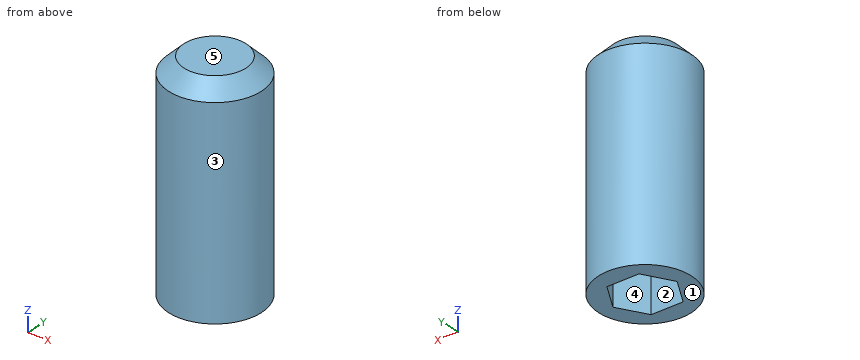
Autodesk Inventor part; units mm, degrees
ref_plane "YZ Plane" through (0, 0, 0) normal (1, 0, 0) x (0, 1, 0)
ref_plane "XZ Plane" through (0, 0, 0) normal (0, 1, 0) x (-1, 0, 0)
ref_plane "XY Plane" through (0, 0, 0) normal (0, 0, 1) x (1, 0, 0)
sketch "Sketch1" plane through (0, 0, 0) normal (0, 0, 1) x (1, 0, 0)
  circle A0 centre (0, 0) radius 1.5
  dimension "d0" = 3
extrude "Extrusion1" add sketch "Sketch1" along normal blind 7
chamfer "Chamfer1" distance 0.5 angle 45 1 edges at (-1.5, 0, 7)
sketch "Sketch2" plane through (0, 0, 0) normal (0, 0, -1) x (-1, 0, 0)
  line L0 (-0.5196, 0.9) -> (0.5196, 0.9)
  line L1 (0.5196, 0.9) -> (1.0392, 0)
  line L2 (1.0392, 0) -> (0.5196, -0.9)
  line L3 (0.5196, -0.9) -> (-0.5196, -0.9)
  line L4 (-0.5196, -0.9) -> (-1.0392, 0)
  line L5 (-1.0392, 0) -> (-0.5196, 0.9)
  point P0 (0, 0)
  point P1 (0, 0)
  dimension "d6" = 1.8
extrude "Extrusion2" cut sketch "Sketch2" against normal blind 2
properties part number "m3_setscrew"
Input: part model. Units: mm. Frame: model coordinates. Face numbers are marked on the shaded views. A direction names the side the tool comes from. Give positions to 0.01 mm unless a question says otherwise; leave off trailing zeros. Write each loop counter-clockwise with the first axis right and the second up, starting at its lowest first coordinate (ties: lowest second). Pieces come first, ordered by that corner, then holes.
Q1. Section C-C, the plane z = 6.75. Output: boundary loops of the cut face in (x, y).
Q2. Material intervals for probe 1 along X at (y, z) = (-0.5, 0.5); probe 2 along Z at (x, y) = (-0.65, 0); probe 3 along Y at (x, z) = (-0.6, 1.75), sorted ascending.
Q3. Set-up query: the marked faces 4 and 5. Return all of +Z, -Z, +X, -X, +Y, -Y with unobstructed straight access to the full face (end or side cutting, diameter ignored); none if empty.
Q4. Section B-B, the plane x = 0. Output: boundary loops of the cut face in (y, z), plus the area to 4 significant figures.
Q5. Section A-A, the plane z = 1. Output: boundary loops of the cut face in (x, y), plus the area to 3 significant figures.
Q6. Section D-D, the plane z = 2.75. Output: boundary loops of the cut face in (x, y), plus the area to 3 significant figures.
Q7. First-contact query: P1, Ø1, axis at y = 1, z = 3, coming from the +X side. Flat tip, straight axial feed; report the tip coordinate or a pass-through.
Q8. Pull-direction query (Y, two-part tool) for the marked faces 1, 2 and 3; classes: pulls with the +Y half, pulls with the -Y half, needs draft (parallel to the pull), parting line crosses it, or undercut.
Filled in:
1. outline: circle Ø2.5 at (0, 0)
2. probe 1: x = -1.41 to -0.75, 0.75 to 1.41
2. probe 2: z = 2 to 7
2. probe 3: y = -1.37 to -0.76, 0.76 to 1.37
3. face 4: -Z
3. face 5: +Z, +X, -X, +Y, -Y
4. outline: (-1.5, 0) - (-0.9, 0) - (-0.9, 2) - (0.9, 2) - (0.9, 0) - (1.5, 0) - (1.5, 6.5) - (1, 7) - (-1, 7) - (-1.5, 6.5) - close
4. area: 17.15 mm2
5. outline: circle Ø3 at (0, 0); hole (-1.04, 0) - (-0.52, -0.9) - (0.52, -0.9) - (1.04, 0) - (0.52, 0.9) - (-0.52, 0.9) - close
5. area: 4.26 mm2
6. outline: circle Ø3 at (0, 0)
6. area: 7.07 mm2
7. P1: stops at x = 1.41
8. face 1: needs draft
8. face 2: undercut
8. face 3: parting line crosses it
